Source: CAD feature listing. Evaluate the final solid. Frame: model axes, mm. A direction names the side the tool comes from. Round coordinates to 2 decimals unless told otherwise and drop trailing zeros. Order: outer loops, then holes, each group sorted by start corner. A loop starts at its lowest first (then second) coordinate and runs counter-clockwise, first axis right, second up. Notation, with made-up numbers: (25.5, 48) -> (56.5, 48) arc R17 ccw to (56.5, 78) -> close; hole circle Ø6 at (36.5, 68.5). An arc over 180 degrees is marked (long way). Answer as CSV lines item,"result".
Autodesk Inventor part; units mm, degrees
ref_plane "YZ Plane" through (0, 0, 0) normal (1, 0, 0) x (0, 1, 0)
ref_plane "XZ Plane" through (0, 0, 0) normal (0, 1, 0) x (-1, 0, 0)
ref_plane "XY Plane" through (0, 0, 0) normal (0, 0, 1) x (1, 0, 0)
sketch "Sketch1" plane through (0, 0, 0) normal (0, 0, 1) x (1, 0, 0)
  line L0 (0, 0) -> (-25.4, 0)
  line L1 (-25.4, 0) -> (-25.4, 25.4)
  line L2 (0, 3.175) -> (-22.225, 3.175)
  line L3 (-22.225, 3.175) -> (-22.225, 25.4)
  line L4 (-22.225, 25.4) -> (-25.4, 25.4)
  line L5 (0, 3.175) -> (0, 0)
  dimension "d0" = 25.4
  dimension "d1" = 25.4
  dimension "d2" = 3.175
extrude "Extrusion1" add sketch "Sketch1" along normal mid plane 698.5
properties part number "27.5 Top L"
1. Line query: L1, parallel to X at y = 7, z = 149.5 (3 decimals); L2, parallel to Y at x = -19, z = -268.5 (3 decimals). Output: solid intervals per line, ascending. Write a range as [from, to].
Results below:
L1,"[-25.4, -22.225]"
L2,"[0, 3.175]"
2. Section query C-C on y = 21.5. Return loops of the section in (x, z) (3 decimals), and give its area (3 significant figures).
Results below:
outline,"(-25.4, -349.25) -> (-22.225, -349.25) -> (-22.225, 349.25) -> (-25.4, 349.25) -> close"
area,"2,220 mm2"
3. Section query A-A on z = -50.5. Return loops of the section in (x, y) (3 decimals), and give its area (3 significant figures).
Results below:
outline,"(-25.4, 0) -> (0, 0) -> (0, 3.175) -> (-22.225, 3.175) -> (-22.225, 25.4) -> (-25.4, 25.4) -> close"
area,"151 mm2"
4. Pin query (flat end, axial travel): pin 1 (11 mm diameter, centred on y = 19, z = -85, fed in from +X) (3 decimals); pin 2 (4 mm diameter, centred on x = -7.5, z = -2.5, fed in from +Y) (3 decimals); pin 3 (1 mm diameter, centred on x = -10, y = 4.5, fed in from +Z). Return the tip coordinate at first contact, or that it passes through.
Results below:
pin 1,"x = -22.225"
pin 2,"y = 3.175"
pin 3,"through"
5. Section query B-B on x = -15. Return loops of the section in (y, z) (3 decimals).
Results below:
outline,"(0, -349.25) -> (3.175, -349.25) -> (3.175, 349.25) -> (0, 349.25) -> close"
6. Reachability of faces 1 (the flat face through (-13, 0, -5)), 2 (the flat face through (-11, 3.175, -5)) from +Z, -Z, +X, -X, +Y, -Y: full face, straight path, thin tool, end or side. Return the list, or none.
Results below:
face 1,"+Z, -Z, +X, -X, -Y"
face 2,"+Z, -Z, +X, +Y"
